```python
from build123d import *

# Parameters (mm, degrees)
SKETCH1_R           = 38.1
SKETCH1_R_2         = 15.875
SKETCH1_R_3         = 2.0193
BOSS_EXTRUDE1_DEPTH = 3.175
BOSS_EXTRUDE2_START = 3.175
SKETCH2_R           = 34.8488
SKETCH2_R_2         = 2.0193
SKETCH2_R_3         = 15.875
BOSS_EXTRUDE2_DEPTH = 3.175
CHAMFER1_SIZE       = 1.5875


with BuildPart() as part:
    # Sketch1 → Boss-Extrude1 (new, symmetric)
    with BuildSketch(Plane(origin=(0, 0, 0), x_dir=(0, 0, -1), z_dir=(1, 0, 0))):
        Circle(SKETCH1_R)
        Circle(SKETCH1_R_2, mode=Mode.SUBTRACT)
        with Locations((11.90625, 20.622229928)):
            Circle(SKETCH1_R_3, mode=Mode.SUBTRACT)
        with Locations((23.8125, 0)):
            Circle(SKETCH1_R_3, mode=Mode.SUBTRACT)
        with Locations((11.90625, -20.622229928)):
            Circle(SKETCH1_R_3, mode=Mode.SUBTRACT)
        with Locations((-11.90625, -20.622229928)):
            Circle(SKETCH1_R_3, mode=Mode.SUBTRACT)
        with Locations((-23.8125, 0)):
            Circle(SKETCH1_R_3, mode=Mode.SUBTRACT)
        with Locations((-11.90625, 20.622229928)):
            Circle(SKETCH1_R_3, mode=Mode.SUBTRACT)
    extrude(amount=BOSS_EXTRUDE1_DEPTH, both=True)

    # Sketch2 → Boss-Extrude2 (add)
    with BuildSketch(Plane.ZY.offset(3.175).offset(BOSS_EXTRUDE2_START)):
        with Locations(Location((0, 0, 0), (0, 0, 270))):
            Circle(SKETCH2_R)
        with Locations(Location((-11.90625, 20.622229928, 0), (0, 0, 270))):
            Circle(SKETCH2_R_2, mode=Mode.SUBTRACT)
        with Locations(Location((-11.90625, -20.622229928, 0), (0, 0, 270))):
            Circle(SKETCH2_R_2, mode=Mode.SUBTRACT)
        with Locations(Location((23.8125, 0, 0), (0, 0, 270))):
            Circle(SKETCH2_R_2, mode=Mode.SUBTRACT)
        with Locations(Location((11.90625, 20.622229928, 0), (0, 0, 270))):
            Circle(SKETCH2_R_2, mode=Mode.SUBTRACT)
        with Locations(Location((11.90625, -20.622229928, 0), (0, 0, 270))):
            Circle(SKETCH2_R_2, mode=Mode.SUBTRACT)
        with Locations(Location((-23.8125, 0, 0), (0, 0, 270))):
            Circle(SKETCH2_R_2, mode=Mode.SUBTRACT)
        with Locations(Location((0, 0, 0), (0, 0, 270))):
            Circle(SKETCH2_R_3, mode=Mode.SUBTRACT)
    extrude(amount=-BOSS_EXTRUDE2_DEPTH)

    # Chamfer1
    chamfer1_edges = [part.edges().sort_by_distance(p)[0] for p in [
        (-3.175, 0, 38.1),
    ]]
    chamfer(chamfer1_edges, length=CHAMFER1_SIZE)


solid = part.part
```
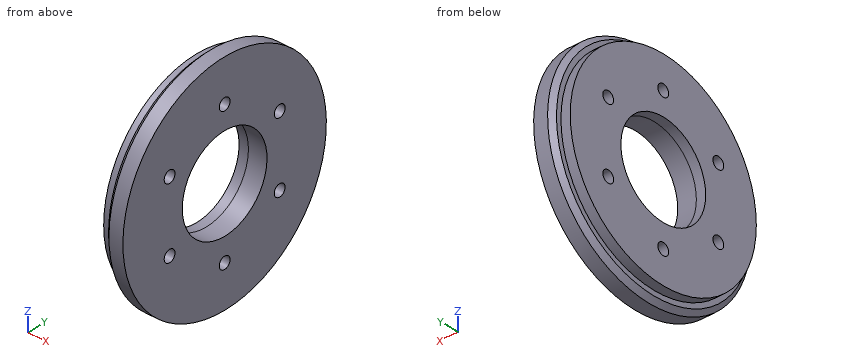
Can you work these out from the model? Positions are in its coordinate system, mm. Round coordinates to 2 decimals unless told otherwise and drop trailing zeros. Answer as a JSON object with one key per item and string values. Group by question number.
Q1. Will these pins go through, and if not, where does the flat tip stop? pin 1 (1 mm diameter, centred on y = 2.5, z = -15, fed in from +X); pin 2 (4.5 mm diameter, centred on y = 0, z = -23.81, fed in from -X); pin 3 (4 mm diameter, centred on x = -3.5, z = -12.5, fed in from -Y).
Q2. Please list where these lines run through material, in increasing order: L1, parallel to Y at x = -4.25, z = 11.5; L2, parallel to Y at x = 2.5, z = -11; L3, parallel to Z at x = -3, y = 19.
Q3. Imagine slicing it at B-B, the plane y = 0. Count the separate pieces of the cut face and the enclosed holes in it, then the cut area to 3 significant figures.
Findings:
{
 "1": {"pin 1": "passes through", "pin 2": "stops at x = -6.35", "pin 3": "stops at y = -36.19"},
 "2": {"L1": "y = -32.9 to -22.6, -18.64 to -10.94, 10.94 to 18.64, 22.6 to 32.9", "L2": "y = -36.48 to -22.43, -18.82 to -11.45, 11.45 to 18.82, 22.43 to 36.48", "L3": "z = -31.38 to -13.11, -10.7 to 10.7, 13.11 to 31.38"},
 "3": {"separate pieces": "4", "enclosed holes": "0", "area": "323 mm2"}
}
